Verification items for the finished model (mm, model axes). Face numbers are marked on the shaded views. A direction names the side the tool comes from. Give positions to 0.01 mm unless a question says otherwise; leave off trailing zeros. Order: outer loops, then holes, each group sorted by start corner. A loop starts at its lowest first (then second) coordinate and runs counter-clockwise, first axis right, second up. Notation, with made-up numbers: (78, 57) - (99, 57) arc R24 cw to (99, 74) - close; hole circle Ø9 at (60.25, 65.25). An arc over 180 degrees is marked (long way). Answer as a JSON object with one key per item and string values. Group by question number.
(1) Section check C-C (y = -0.45). Record the boundary of the cut face in (x, z), then the cut area to 4 significant figures.
(2) Thickness scan on line 1 (Z direction, x = -2.25, y = -0.05); line 2 (Y direction, x = -1.5, z = 8.5); line 3 (X direction, y = 2.4, z = 25.5). Record the ranges inside material, lowest first.
(3) Section check A-A (x = 2). Record the boundary of the cut face in (y, z).
(4) Depth check by flat-ended pin: pin 1 Ø1 at (y, z) = (-0.5, 6) entering from +X; pin 2 Ø4 at (x, z) = (5.5, 23) entering from -Y; pin 3 Ø1.6 at (x, y) = (5, -0.5) entering from +Z. Enter the tip coordinate at first touch or a pass-through.
(5) Access from +Z, -Z, +X, -X, +Y, -Y to the whole of each face (thin tool, end or side, straight path). Record for the marked faces 1 and 2.
(6) Section check B-B (z = 25). Record the boundary of the cut face in (x, y), then the cut area to 4 significant figures.
(7) Section check D-D (z = 4.5). Record the boundary of the cut face in (x, y).
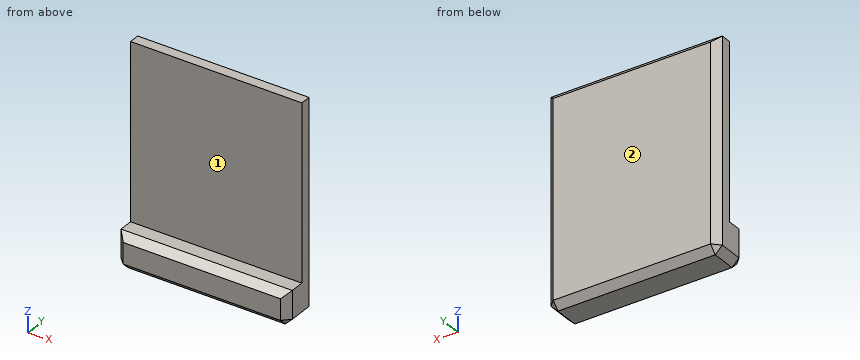
```python
from build123d import *

# Parameters (mm, degrees)
SKETCH006_W  = 24.5
SKETCH006_H  = 2.5
PAD003_DEPTH = 30
SKETCH007_W  = 24.5
SKETCH007_H  = 5
PAD004_DEPTH = 3
CHAMFER_SIZE = 1


with BuildPart() as part:
    # Sketch006 (on XY_Plane003 of Origin006) → Pad003 (new body)
    with BuildSketch(Plane.XY):
        with Locations((5.368647, 1.814191)):
            Rectangle(SKETCH006_W, SKETCH006_H)
    extrude(amount=PAD003_DEPTH)

    # Sketch007 (on Face1 of Pad003) → Pad004 (join)
    with BuildSketch(Plane.XZ.offset(-0.564191)):
        with Locations((5.368647, 2.5)):
            Rectangle(SKETCH007_W, SKETCH007_H)
    extrude(amount=PAD004_DEPTH)

    # Chamfer
    chamfer_edges = [part.edges().sort_by_distance(p)[0] for p in [
        (17.618647, -2.435809, 2.5),
        (5.368647, -2.435809, 5),
        (-6.881353, -2.435809, 2.5),
        (5.368647, -2.435809, 0),
        (17.618647, 0.314191, 0),
        (-6.881353, 0.314191, 0),
        (5.368647, 3.064191, 0),
        (17.618647, 3.064191, 15),
        (-6.881353, 3.064191, 15),
        (5.368647, 3.064191, 30),
    ]]
    chamfer(chamfer_edges, length=CHAMFER_SIZE)


solid = part.part
```
Solutions:
{
 "1": {"outline": "(-6.88, 1) - (-5.88, 0) - (16.62, 0) - (17.62, 1) - (17.62, 5) - (-6.88, 5) - close", "area": "121.5 mm2"},
 "2": {"line 1": "z = 0 to 5", "line 2": "y = 0.56 to 3.06", "line 3": "x = -6.55 to 17.28"},
 "3": {"outline": "(-2.44, 1) - (-1.44, 0) - (2.06, 0) - (3.06, 1) - (3.06, 29) - (2.06, 30) - (0.56, 30) - (0.56, 5) - (-1.44, 5) - (-2.44, 4) - close"},
 "4": {"pin 1": "passes through", "pin 2": "stops at y = 0.56", "pin 3": "stops at z = 5"},
 "5": {"face 1": "+Z, +X, -X, -Y", "face 2": "+Z, -Z, +X, -X, +Y"},
 "6": {"outline": "(-6.88, 0.56) - (17.62, 0.56) - (17.62, 2.06) - (16.62, 3.06) - (-5.88, 3.06) - (-6.88, 2.06) - close", "area": "60.25 mm2"},
 "7": {"outline": "(-6.88, -1.44) - (-6.38, -1.94) - (17.12, -1.94) - (17.62, -1.44) - (17.62, 2.06) - (16.62, 3.06) - (-5.88, 3.06) - (-6.88, 2.06) - close"}
}
